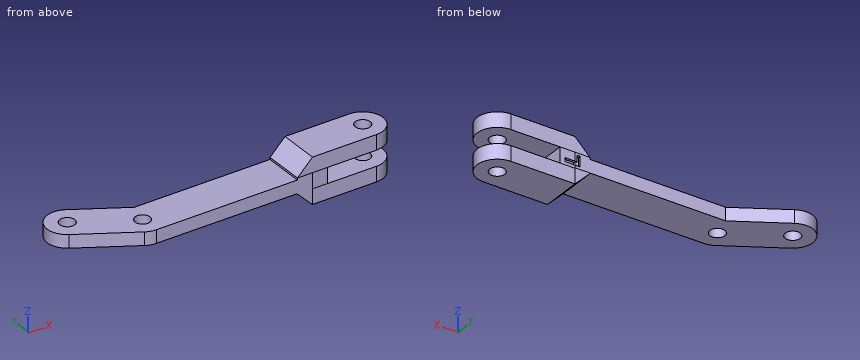
Autodesk Inventor part; units mm, degrees
ref_plane "Work Plane1" through (-62.942605, 1.312432, -0.38873) normal (0, 0, -1) x (-0.0504539, 0.9987264, 0)
ref_plane "YZ Plane" through (0, 0, 0) normal (1, 0, 0) x (0, 1, 0)
ref_plane "XZ Plane" through (0, 0, 0) normal (0, 1, 0) x (-1, 0, 0)
sketch "Sketch1" plane through (0, 0, 0) normal (0, 0, 1) x (1, 0, 0)
  line L0 (-26.293304, 15.205533) -> (-26.696935, 23.195344)
  line L1 (-26.696935, 23.195344) -> (-13.921595, 23.840732)
  arc A0 (-13.517964, 15.85092) -> (-13.921595, 23.840732) centre (-13.719779, 19.845826) ccw
  line L2 (-13.517964, 15.85092) -> (-26.293304, 15.205533)
  circle A1 centre (-13.719779, 19.845826) radius 1.5
  point P0 (0, 0)
sketch "Sketch1 outline for Extrusion1" plane through (0, 0, 0) normal (0, 0, 1) x (1, 0, 0)
  arc A0 (-13.517964, 15.85092) -> (-13.921595, 23.840732) centre (-13.719779, 19.845826) ccw
  line L0 (-26.293304, 15.205533) -> (-13.517964, 15.85092)
  line L1 (-13.921595, 23.840732) -> (-26.696935, 23.195344)
  line L2 (-26.696935, 23.195344) -> (-26.293304, 15.205533)
  circle A1 centre (-13.719779, 19.845826) radius 1.5
extrude "Extrusion1" add sketch "Sketch1 outline for Extrusion1" along normal blind 3
sketch "Sketch2" plane through (0, 0, 0) normal (0, 0, -1) x (-1, 0, 0)
  line L0 (23.700756, 23.346705) -> (23.297124, 15.356894)
  line L1 (26.696935, 23.195344) -> (26.293304, 15.205533)
  line L2 (13.921595, 23.840732) -> (26.696935, 23.195344)
  arc A0 (13.921595, 23.840732) -> (13.517964, 15.85092) centre (13.719779, 19.845826) ccw
  line L3 (26.293304, 15.205533) -> (13.517964, 15.85092)
  line L4 (26.696935, 23.195344) -> (26.293304, 15.205533)
  circle A1 centre (13.719779, 19.845826) radius 1.5
  point P0 (0, 0)
sketch "Sketch2 outline for Extrusion2" plane through (0, 0, 0) normal (0, 0, -1) x (-1, 0, 0)
  line L0 (23.297124, 15.356894) -> (26.293304, 15.205533)
  line L1 (23.700756, 23.346705) -> (23.297124, 15.356894)
  line L2 (26.696935, 23.195344) -> (23.700756, 23.346705)
  line L3 (26.293304, 15.205533) -> (26.696935, 23.195344)
extrude "Extrusion2" add sketch "Sketch2 outline for Extrusion2" along normal blind 3.1
sketch "Sketch3" plane through (0, 0, -3.1) normal (0, 0, -1) x (-1, 0, 0)
  line L0 (13.921595, 23.840732) -> (26.696935, 23.195344)
  line L1 (26.696935, 23.195344) -> (26.293304, 15.205533)
  line L2 (26.293304, 15.205533) -> (13.517964, 15.85092)
  arc A0 (13.921595, 23.840732) -> (13.517964, 15.85092) centre (13.719779, 19.845826) ccw
  circle A1 centre (13.719779, 19.845826) radius 1.5
  point P0 (0, 0)
sketch "Sketch3 outline for Extrusion3" plane through (0, 0, -3.1) normal (0, 0, -1) x (-1, 0, 0)
  arc A0 (13.921595, 23.840732) -> (13.517964, 15.85092) centre (13.719779, 19.845826) ccw
  line L0 (26.696935, 23.195344) -> (13.921595, 23.840732)
  line L1 (13.517964, 15.85092) -> (26.293304, 15.205533)
  line L2 (26.293304, 15.205533) -> (26.696935, 23.195344)
  circle A1 centre (13.719779, 19.845826) radius 1.5
extrude "Extrusion3" add sketch "Sketch3 outline for Extrusion3" along normal blind 3
sketch "Sketch4" plane through (0, 0, 0) normal (0, 0, -1) x (-1, 0, 0)
  arc A0 (57.453567, 13.631371) -> (57.857198, 21.621182) centre (57.655383, 17.626276) ccw
  line L0 (57.453567, 13.631371) -> (29.389355, 15.049125)
  line L1 (29.792987, 23.038937) -> (29.389355, 15.049125)
  line L2 (29.792987, 23.038937) -> (57.857198, 21.621182)
  circle A1 centre (57.655383, 17.626276) radius 1.5
  line L3 (29.389355, 15.049125) -> (26.293304, 15.205533)
  line L4 (26.696935, 23.195344) -> (26.293304, 15.205533)
  line L5 (26.696935, 23.195344) -> (29.792987, 23.038937)
  line L6 (29.792987, 23.038937) -> (29.389355, 15.049125)
  circle A2 centre (68.688702, 23.388615) radius 1.5
  arc A3 (70.540437, 19.843043) -> (66.836967, 26.934186) centre (68.688702, 23.388615) ccw
  line L7 (59.507118, 14.080705) -> (70.540437, 19.843043)
  arc A4 (57.453567, 13.631371) -> (57.857198, 21.621182) centre (57.655383, 17.626276) ccw
  line L8 (56.769238, 21.676144) -> (66.836967, 26.934186)
  point P0 (0, 0)
  dimension "d18" = 8
sketch "Sketch4 outline for Extrusion4" plane through (0, 0, 0) normal (0, 0, -1) x (-1, 0, 0)
  line L0 (26.696935, 23.195344) -> (26.293304, 15.205533)
  line L1 (26.293304, 15.205533) -> (57.453567, 13.631371)
  arc A0 (57.453567, 13.631371) -> (59.507118, 14.080705) centre (57.655383, 17.626276) ccw
  line L2 (59.507118, 14.080705) -> (70.540437, 19.843043)
  arc A1 (70.540437, 19.843043) -> (66.836967, 26.934186) centre (68.688702, 23.388615) ccw
  line L3 (66.836967, 26.934186) -> (56.769238, 21.676144)
  line L4 (56.769238, 21.676144) -> (26.696935, 23.195344)
  circle A2 centre (57.655383, 17.626276) radius 1.5
  circle A3 centre (68.688702, 23.388615) radius 1.5
extrude "Extrusion4" add sketch "Sketch4 outline for Extrusion4" along normal blind 3
chamfer "Chamfer1" distance 3 angle 45 1 edges at (-26.4951, 19.2004, 0)
chamfer "Chamfer2" distance 3.1 angle 45 1 edges at (-26.4951, 19.2004, -3)
ref_plane "Work Plane1" through (-62.942605, 1.312432, -0.38873) normal (0, 0, -1) x (-0.0504539, 0.9987264, 0)
sketch "Sketch6" plane through (0, 0, 0) normal (0, 0, 1) x (1, 0, 0)
  line L0 (-57.453567, 13.631371) -> (-48.265284, 14.095547)
  arc A0 (-57.857198, 21.621182) -> (-57.453567, 13.631371) centre (-57.655383, 17.626276) ccw
  line L1 (-29.693114, 23.043982) -> (-57.857198, 21.621182)
  line L2 (-29.693114, 23.043982) -> (-48.265284, 14.095547)
  circle A1 centre (-57.655383, 17.626276) radius 1.5
  point P0 (0, 0)
sketch "Sketch6 outline for Extrusion5" plane through (0, 0, 0) normal (0, 0, 1) x (1, 0, 0)
  line L0 (-29.693114, 23.043982) -> (-57.857198, 21.621182)
  line L1 (-48.265284, 14.095547) -> (-29.693114, 23.043982)
  arc A0 (-57.857198, 21.621182) -> (-57.453567, 13.631371) centre (-57.655383, 17.626276) ccw
  line L2 (-57.453567, 13.631371) -> (-48.265284, 14.095547)
  circle A1 centre (-57.655383, 17.626276) radius 1.5
extrude "Extrusion5" cut sketch "Sketch6 outline for Extrusion5" against normal up to surface (0.38873 mm away)
sketch "Sketch7" plane through (-13.921595, 23.840732, 3) normal (-0.0504539, 0.9987264, 0) x (0.9987264, 0.0504539, 0)
  line L0 (-10.748057, 5.806776) -> (-10.748057, 3.406816) construction
  line L1 (-10.748057, 3.406816) -> (-13.798057, 3.406816) construction
  line L2 (-13.798057, 3.406816) -> (-13.798057, 5.806776) construction
  line L3 (-13.798057, 5.806776) -> (-10.748057, 5.806776) construction
  line L4 (-13.798057, 3.456249) -> (-13.798057, 5.490406)
  line L5 (-13.798057, 5.490406) -> (-10.748057, 5.490406)
  line L6 (-10.748057, 5.490406) -> (-10.748057, 4.724199)
  line L7 (-10.748057, 4.724199) -> (-13.217222, 4.724199)
  line L8 (-13.217222, 4.724199) -> (-13.217222, 3.456249)
  line L9 (-13.217222, 3.456249) -> (-13.798057, 3.456249)
  point P0 (12.701006, 3)
sketch "Sketch7 outline for Emboss1" plane through (-13.921595, 23.840732, 3) normal (-0.0504539, 0.9987264, 0) x (0.9987264, 0.0504539, 0)
  line L0 (-13.798057, 3.456249) -> (-13.798057, 5.490406)
  line L1 (-13.798057, 5.490406) -> (-10.748057, 5.490406)
  line L2 (-10.748057, 5.490406) -> (-10.748057, 4.724199)
  line L3 (-10.748057, 4.724199) -> (-13.217222, 4.724199)
  line L4 (-13.217222, 4.724199) -> (-13.217222, 3.456249)
  line L5 (-13.217222, 3.456249) -> (-13.798057, 3.456249)
emboss "Emboss1" sketch "Sketch7 outline for Emboss1" operation cut depth 0.5 direction (0.0504539, -0.9987264, 0)
sketch "Sketch8" plane through (0, 0, 0) normal (0, 0, 1) x (1, 0, 0)
  line L0 (-57.857198, 21.621182) -> (-56.769238, 21.676144)
  line L1 (-66.836967, 26.934186) -> (-56.769238, 21.676144)
  arc A0 (-66.836967, 26.934186) -> (-70.540437, 19.843043) centre (-68.688702, 23.388615) ccw
  line L2 (-59.507118, 14.080705) -> (-70.540437, 19.843043)
  arc A1 (-57.857198, 21.621182) -> (-59.507118, 14.080705) centre (-57.655383, 17.626276) ccw
  circle A2 centre (-68.688702, 23.388615) radius 1.5
  point P0 (0, 0)
sketch "Sketch8 outline for Extrusion6" plane through (0, 0, 0) normal (0, 0, 1) x (1, 0, 0)
  arc A0 (-59.507118, 14.080705) -> (-57.857198, 21.621182) centre (-57.655383, 17.626276) cw
  line L0 (-70.540437, 19.843043) -> (-59.507118, 14.080705)
  line L1 (-57.857198, 21.621182) -> (-56.769238, 21.676144)
  arc A1 (-66.836967, 26.934186) -> (-70.540437, 19.843043) centre (-68.688702, 23.388615) ccw
  line L2 (-56.769238, 21.676144) -> (-66.836967, 26.934186)
  circle A2 centre (-68.688702, 23.388615) radius 1.5
extrude "Extrusion6" cut sketch "Sketch8 outline for Extrusion6" against normal up to surface (0.38873 mm away)
sketch "Sketch9" plane through (0, 0, 0) normal (0, 0, 1) x (1, 0, 0)
  line L0 (-29.693114, 23.043982) -> (-48.265284, 14.095547)
  line L1 (-29.289483, 15.054171) -> (-48.265284, 14.095547)
  line L2 (-29.693114, 23.043982) -> (-29.289483, 15.054171)
  point P0 (0, 0)
sketch "Sketch9 outline for Extrusion7" plane through (0, 0, 0) normal (0, 0, 1) x (1, 0, 0)
  line L0 (-29.289483, 15.054171) -> (-29.693114, 23.043982)
  line L1 (-48.265284, 14.095547) -> (-29.289483, 15.054171)
  line L2 (-29.693114, 23.043982) -> (-48.265284, 14.095547)
extrude "Extrusion7" cut sketch "Sketch9 outline for Extrusion7" against normal up to surface (0.38873 mm away)
properties part number "GripperShaftLeft_3DPrint"
For this review, take the finished solid that the model builds, in its own axes (mm). Coordinates: 2 decimals unless noted, no trailing zeros. Write each loop counter-clockwise with the first axis right and the second up, starting at its lowest first coordinate (ties: lowest second). Pieces come first, ordered by that corner, then holes. Notation, with made-up numbers: (-17.75, -23.75) -> (-2.75, -23.75) arc R24 cw to (-2.75, -3.75) -> close; hole circle Ø3 at (20, 72). An arc over 180 degrees is marked (long way). Put each result on its own line as item: value.
Q1. Take a section at A-A, the plane x = -22.5. State the section outline as (y, z) points.
From the geometry:
outline: (15.4, -6.1) -> (23.41, -6.1) -> (23.41, -3.1) -> (15.4, -3.1) -> close; (15.4, 0) -> (23.41, 0) -> (23.41, 3) -> (15.4, 3) -> close
Q2. Take a section at D-D, the plane x = -49.5. State the section outline as (y, z) points.
From the geometry:
outline: (14.03, -3) -> (22.04, -3) -> (22.04, -0.39) -> (14.03, -0.39) -> close
Q3. Take a section at B-B, the plane z = -4.75. State the section outline as (x, y) points, then the cut area to 3 significant figures.
From the geometry:
outline: (-28.05, 23.13) -> (-27.64, 15.14) -> (-13.52, 15.85) arc R4 ccw to (-13.92, 23.84) -> close; hole circle Ø3 at (-13.72, 19.85)
area: 131 mm2
Q4. Wall thickness on L1, parallel to Z at x = -21, y = 18.5; L2, parallel to Z at x = -48, y = 15.5; L3, parallel to X at y = 18, z = -1.5: over which ranges is each line inside the solid? List them lowest first.
From the geometry:
L1: z = -6.1 to -3.1, 0 to 3
L2: z = -3 to -0.39
L3: x = -67.01 to -59.11, -56.2 to -23.43
Q5. Clearance check with flat-ended pins moving along their axes: pin 1 Ø3 at (x, z) = (-41, -2) entering from +Y; pin 2 Ø3.5 at (x, y) = (-57.66, 17.63) entering from -Z; pin 3 Ø2 at (x, y) = (-61, 18) entering from +Z; pin 4 Ø1.8 at (x, y) = (-13.72, 19.85) entering from +Z. State where each tip first meets the part, or that it passes through.
From the geometry:
pin 1: stops at y = 22.55
pin 2: stops at z = -3
pin 3: stops at z = -0.39
pin 4: passes through
Q6. Take a section at C-C, the plane z = 1.5. State the section outline as (x, y) points, then the cut area to 3 significant figures.
From the geometry:
outline: (-28.19, 23.12) -> (-27.79, 15.13) -> (-13.52, 15.85) arc R4 ccw to (-13.92, 23.84) -> close; hole circle Ø3 at (-13.72, 19.85)
area: 132 mm2
